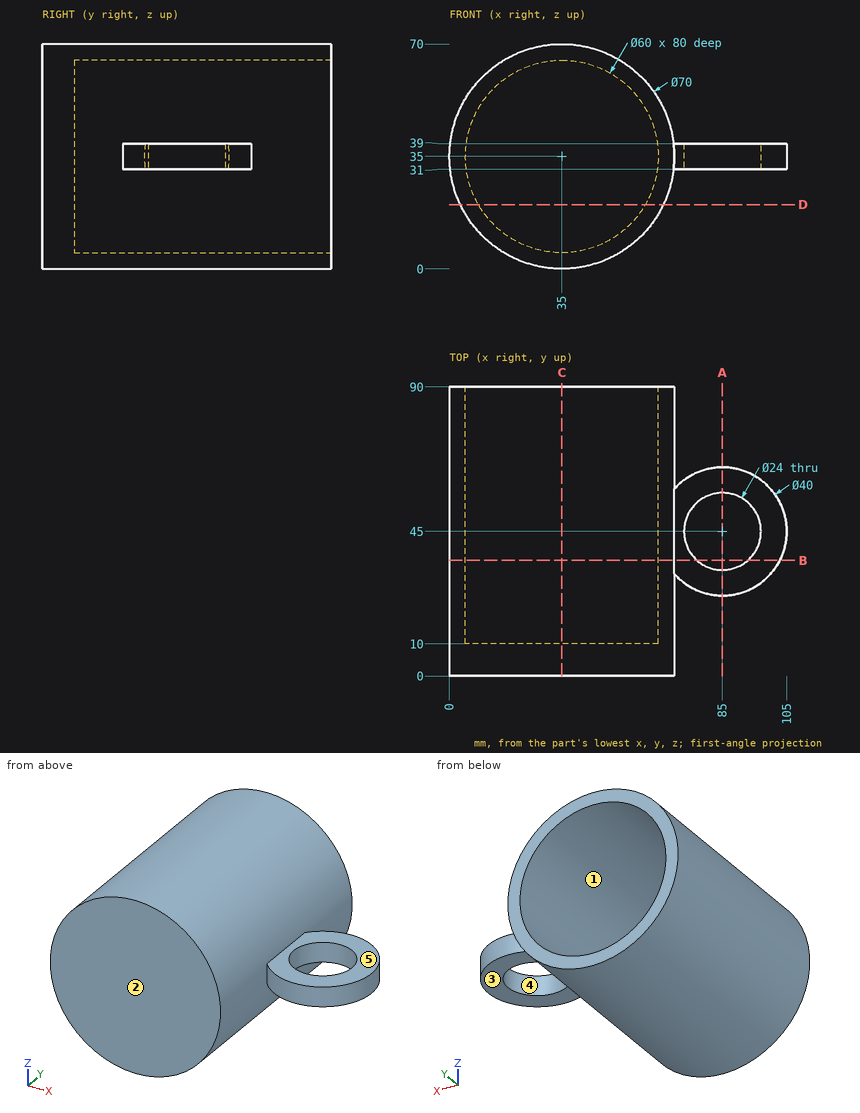
Geometry: see drawing. Coordinates: mm, zero at the bounding-box minimum. A direction names the side the tool comes from. Give positions to 0.01 mm unless a question says otherwise; leave off trailing zeros. Write each loop counter-clockwise with the first axis right and the second up, starting at its lowest first coordinate (ties: lowest second). Pieces come first, ordered by that corner, then holes. Notation, with made-up numbers: M 27,-30 L 40,-30 A22 cw 40,8 Z; hole C 22,-16 d3. An arc over 180 degrees is marked long. Answer in a Markdown table with one row per item. Add a question column.
(1) Reachability of the marked faces 3, 4 and 5 from +Z, -Z, +X, -X, +Y, -Y: full face, straight path, thin tool, end or side. Return the list, or none.
(2) Section D-D on z = 20. Return loops of the section in (x, y), and give its area (3 significant figures).
(3) Section A-A on x = 85. Return loops of the section in (y, z), and give its area (3 significant figures).
(4) Ray query, line 1 (Y direction, x = 85, z = 34.75); line 2 (Y direction, x = 61.5, z = 42); line 3 (X direction, y = 82.5, z = 61.5). Return the intervals inside material, ascending.
(5) Section B-B on y = 36. Return loops of the section in (x, z), and give its area (3 significant figures).
(6) First-contact query: pin 1 (5 mm diameter, centred on y = 55, z = 60.5, fed in from +X); pin 2 (5 mm diameter, centred on y = 44.5, z = 46.5, fed in from +X); pin 3 (1.5 mm diameter, centred on x = 63, y = 31, fed in from +Z); pin 4 (14.5 mm diameter, centred on x = 85, y = 45, fed in from -Z). Flat tips, straight axial feed; report the tip coordinate or a pass-through.
(7) Mould query, pull axis X, two halves, no side actions, for the marked faces 1 and 2. Classes: +X half, -X half, draft (parallel to the pull), parting line (faces both ways), or undercut.
(8) Section C-C on x = 35. Return loops of the section in (y, z), and give its area (3 significant figures).
Result set:
| question | item | result |
|---|---|---|
| 1 | face 3 | -Z, +X, +Y, -Y |
| 1 | face 4 | +Z, -Z |
| 1 | face 5 | +Z, +X, +Y, -Y |
| 2 | outline | M 3.38,0 L 66.62,0 L 66.62,90 L 60.98,90 L 60.98,10 L 9.02,10 L 9.02,90 L 3.38,90 Z |
| 2 | area | 1,540 mm^2 |
| 3 | outline | M 25,31 L 33,31 L 33,39 L 25,39 Z; M 57,31 L 65,31 L 65,39 L 57,39 Z |
| 3 | area | 128 mm^2 |
| 4 | line 1 | y = 25 to 33, 57 to 65 |
| 4 | line 2 | y = 0 to 10 |
| 4 | line 3 | x = 12.14 to 20.94, 49.06 to 57.86 |
| 5 | outline | M 69.77,31 L 77.06,31 L 77.06,39 L 69.77,39 A35 ccw long Z; M 92.94,31 L 102.86,31 L 102.86,39 L 92.94,39 Z; hole C 35,35 d60 |
| 5 | area | 1,160 mm^2 |
| 6 | pin 1 | stops at x = 61.38 |
| 6 | pin 2 | stops at x = 68.82 |
| 6 | pin 3 | stops at z = 56.96 |
| 6 | pin 4 | passes through |
| 7 | face 1 | undercut |
| 7 | face 2 | draft |
| 8 | outline | M 0,0 L 90,0 L 90,5 L 10,5 L 10,65 L 90,65 L 90,70 L 0,70 Z |
| 8 | area | 1,500 mm^2 |
